The model under review builds one solid part; all positions refer to its coordinate system, in mm. A direction names the side the tool comes from. Give positions to 0.01 mm unless a question says otherwise; leave off trailing zeros. Loops run counter-clockwise (first coordinate to the right, second up) from the corner with the lowest first, then second, coordinate; pieces in that order, holes last. Notation, with made-up numbers: M 23,52.25 L 52,52.25 A23 ccw 52,86.25 Z; hole C -34.75,-28.5 d2. An arc over 180 degrees is marked long. Return JSON: item names as keys, results as strings.
```python
from build123d import *

# Parameters (mm, degrees)
BOSS_EXTRUDE4_DEPTH   = 5
BOSS_EXTRUDE4_2_DEPTH = 5
SKETCH3_W             = 13
SKETCH3_H             = 13
CUT_EXTRUDE2_DEPTH    = 126.39936204
BOSS_EXTRUDE5_DEPTH   = 5
BOSS_EXTRUDE6_START   = 50
BOSS_EXTRUDE6_DEPTH   = 5
SKETCH5_W             = 5
SKETCH5_H             = 30
BOSS_EXTRUDE7_DEPTH   = 40
SKETCH6_R             = 3
CUT_EXTRUDE3_DEPTH    = 110.658560997


with BuildPart() as part:
    # Sketch1 → Boss-Extrude4 (new body)
    with BuildSketch(Plane.XY):
        Polygon((0, 0), (50, 0), (60, 10), (60, 30), (0, 30), align=None)
    extrude(amount=BOSS_EXTRUDE4_DEPTH)


with BuildPart() as body_2:
    # Sketch1 → Boss-Extrude4 2 (new body)
    with BuildSketch(Plane.XY):
        Polygon((0, 80), (0, 110), (50, 110), (60, 100), (60, 80), align=None)
    extrude(amount=BOSS_EXTRUDE4_2_DEPTH)


with BuildPart() as cut_extrude2_tool:
    # Sketch3 → Cut-Extrude2 (new, through all)
    with BuildSketch(Plane.XY.offset(5)):
        with Locations((13, 97)):
            Rectangle(SKETCH3_W, SKETCH3_H)
        with Locations((38, 97)):
            Rectangle(SKETCH3_W, SKETCH3_H)
        with Locations((13, 13)):
            Rectangle(SKETCH3_W, SKETCH3_H)
        with Locations((38, 13)):
            Rectangle(SKETCH3_W, SKETCH3_H)
    extrude(amount=-CUT_EXTRUDE2_DEPTH)


with BuildPart() as part_1:
    add(part.part)

    # Cut-Extrude2: cut by cut_extrude2_tool
    add(cut_extrude2_tool.part, mode=Mode.SUBTRACT)

    # Sketch4 → Boss-Extrude5 (add)
    with BuildSketch(Plane(origin=(0, 30, 0), x_dir=(1, 0, 0), z_dir=(0, 1, 0))):
        Polygon((60, -5), (60, -11), (38, -45), (0, -45), (0, -15), (13, -15), (13, -5), (13, 0), (60, 0), align=None)
    extrude(amount=BOSS_EXTRUDE5_DEPTH)



with BuildPart() as body_2_1:
    add(body_2.part)

    # Cut-Extrude2: cut by cut_extrude2_tool
    add(cut_extrude2_tool.part, mode=Mode.SUBTRACT)

    # Sketch4<2> → Boss-Extrude6 (add)
    with BuildSketch(Plane(origin=(0, 30, 0), x_dir=(1, 0, 0), z_dir=(0, 1, 0)).offset(BOSS_EXTRUDE6_START)):
        Polygon((60, -5), (60, -11), (38, -45), (0, -45), (0, -15), (13, -15), (13, -5), (13, 0), (60, 0), align=None)
    extrude(amount=-BOSS_EXTRUDE6_DEPTH)


with BuildPart() as part_2:
    add(part_1.part)

    add(body_2_1.part)  # Boss-Extrude7 merges body 2
    # Sketch5 → Boss-Extrude7 (add)
    with BuildSketch(Plane(origin=(0, 35, 0), x_dir=(1, 0, 0), z_dir=(0, 1, 0))):
        with Locations((2.5, -30)):
            Rectangle(SKETCH5_W, SKETCH5_H)
    extrude(amount=BOSS_EXTRUDE7_DEPTH)

    # Sketch6 → Cut-Extrude3 (cut, through all)
    with BuildSketch(Plane(origin=(0, 80, 0), x_dir=(1, 0, 0), z_dir=(0, 1, 0))):
        with Locations(Location((20, -35, 0), (0, 0, 180))):
            Circle(SKETCH6_R)
    extrude(amount=-CUT_EXTRUDE3_DEPTH, mode=Mode.SUBTRACT)


solid = part_2.part
```
1) Consider section B-B on z = 12.5. Write out the cut boundary in (x, y).
From the geometry:
{"outline": "M 13,30 L 59.03,30 L 59.03,35 L 13,35 Z; M 13,75 L 59.03,75 L 59.03,80 L 13,80 Z"}
2) Consider section D-D on z = 42. Write out the cut boundary in (x, y).
From the geometry:
{"outline": "M 0,30 L 39.94,30 L 39.94,35 L 5,35 L 5,75 L 39.94,75 L 39.94,80 L 0,80 Z"}
3) Consider section C-C on y = 27.5. Write out the cut boundary in (x, z).
From the geometry:
{"outline": "M 0,0 L 60,0 L 60,5 L 0,5 Z"}
4) Tool access review of faces 4 (the face through (13, 32, 7)), 5 (the face through (30, 15, 5)), 6 (the face through (19.5, 13, 3)): name each direction out of +Z, -Z, +X, -X, +Y, -Y from which nothing blocks a thin tool from reaching the whole face with its end or side.
From the geometry:
{"face 4": "-Z, -X", "face 5": "+Z, +X, -X, -Y", "face 6": "+Z, -Z"}
5) Consider section A-A on z = 33.5. Write out the cut boundary in (x, y), then the cut area to 3 significant figures.
From the geometry:
{"outline": "M 0,30 L 17.4,30 L 17.4,35 L 5,35 L 5,75 L 17.4,75 L 17.4,80 L 0,80 Z; M 22.6,30 L 45.44,30 L 45.44,35 L 22.6,35 Z; M 22.6,75 L 45.44,75 L 45.44,80 L 22.6,80 Z", "area": "602 mm²"}
6) The part is to be moulded in two halves that separate along Y. For faces 1 (the face through (6.5, 13, 3)), 2 (the face through (60, 25, 3)), 3 (the face through (55, 105, 2)), say which applies: released by +Y, released by -Y, zero draft, split by the parting line, or undercut.
From the geometry:
{"face 1": "undercut", "face 2": "zero draft", "face 3": "released by +Y"}
7) Insertion check: pin 1 (5.5 mm diameter, centred on y = 33, z = 10.5, fed in from -X); pin 2 (2 mm diameter, centred on x = 29.5, y = 97.5, fed in from +Z); pin 3 (6 mm diameter, centred on x = 18, z = 8.5, fed in from -Y). Each pin has a flat end and moves straight along its axis. Give the tip position at first contact, or say it passes through.
From the geometry:
{"pin 1": "x = 13", "pin 2": "z = 5", "pin 3": "y = 30"}
8) Wall thickness on L1, parallel to Y at x = 38, z = 4.5; L2, parallel to Z at x = 20, y = 78.9; L3, parallel to Y at x = 35, z = 8.5: over which ranges is each line inside the solid? List them lowest first. Write a range as from..to.
From the geometry:
{"L1": "0..6.5, 19.5..35, 75..90.5, 103.5..110", "L2": "0..32, 38..45", "L3": "30..35, 75..80"}
